The model under review builds one solid part; all positions refer to its coordinate system, in mm. A direction names the side the tool comes from. Give positions to 0.01 mm unless a question says otherwise; leave off trailing zeros. Order: outer loops, then holes, each group sorted by start corner. A loop starts at its lowest first (then second) coordinate and runs counter-clockwise, first axis right, second up. Notation, with made-up numbers: (21.5, 21) - (72.5, 21) arc R26 cw to (72.5, 50) - close; hole circle Ø4 at (65, 9). An arc over 180 degrees is marked (long way). Put each result on its own line as item: value.
```python
from build123d import *

# Parameters (mm, degrees)
CROQUIS1_R              = 25
SALIENTE_EXTRUIR1_DEPTH = 3
CROQUIS2_W              = 12.95
CROQUIS2_H              = 12.95
SALIENTE_EXTRUIR2_DEPTH = 3
CROQUIS3_R              = 2
CORTAR_EXTRUIR1_DEPTH   = 124.455998815
CROQUIS4_R              = 1.5
CORTAR_EXTRUIR2_DEPTH   = 124.455998815


with BuildPart() as part:
    # Croquis1 → Saliente-Extruir1 (new body)
    with BuildSketch(Plane.XY):
        with BuildLine():
            Line((-15.070986718, 74.306476298), (-15.070986718, 37.256476298))
            ThreePointArc((-15.070986718, 37.256476298), (-28.445175059, 28.391049341), (-37.285113206, 15))
            Line((-37.285113206, 15), (-74.335113206, 15))
            Line((-74.335113206, 15), (-74.335113206, 20.59))
            Line((-74.335113206, 20.59), (-87.285113206, 20.59))
            Line((-87.285113206, 20.59), (-87.285113206, -20.59))
            Line((-87.285113206, -20.59), (-74.335113206, -20.59))
            Line((-74.335113206, -20.59), (-74.335113206, -15))
            Line((-74.335113206, -15), (-37.285113206, -15))
            ThreePointArc((-37.285113206, -15), (-28.445175059, -28.391049341), (-15.070986718, -37.256476298))
            Line((-15.070986718, -37.256476298), (-15.070986718, -74.306476298))
            Line((-15.070986718, -74.306476298), (-20.660986718, -74.306476298))
            Line((-20.660986718, -74.306476298), (-20.660986718, -87.256476298))
            Line((-20.660986718, -87.256476298), (20.519013282, -87.256476298))
            Line((20.519013282, -87.256476298), (20.519013282, -74.306476298))
            Line((20.519013282, -74.306476298), (14.929013282, -74.306476298))
            Line((14.929013282, -74.306476298), (14.929013282, -37.256476298))
            ThreePointArc((14.929013282, -37.256476298), (28.353570497, -28.407666286), (37.22795272, -15))
            Line((37.22795272, -15), (59.27795272, -15))
            Line((59.27795272, -15), (59.27795272, -20.59))
            Line((59.27795272, -20.59), (72.22795272, -20.59))
            Line((72.22795272, -20.59), (72.22795272, 20.59))
            Line((72.22795272, 20.59), (59.27795272, 20.59))
            Line((59.27795272, 20.59), (59.27795272, 15))
            Line((59.27795272, 15), (37.22795272, 15))
            ThreePointArc((37.22795272, 15), (28.353570497, 28.407666286), (14.929013282, 37.256476298))
            Line((14.929013282, 37.256476298), (14.929013282, 74.306476298))
            Line((14.929013282, 74.306476298), (20.519013282, 74.306476298))
            Line((20.519013282, 74.306476298), (20.519013282, 87.256476298))
            Line((20.519013282, 87.256476298), (-20.660986718, 87.256476298))
            Line((-20.660986718, 87.256476298), (-20.660986718, 74.306476298))
            Line((-20.660986718, 74.306476298), (-15.070986718, 74.306476298))
        make_face()
        Circle(CROQUIS1_R, mode=Mode.SUBTRACT)
    extrude(amount=SALIENTE_EXTRUIR1_DEPTH)

    # Croquis2 → Saliente-Extruir2 (add)
    with BuildSketch(Plane(origin=(0, 0, 0), x_dir=(-1, 0, 0), z_dir=(0, 0, -1))):
        with Locations((-26.994013282, 80.781476298)):
            Rectangle(CROQUIS2_W, CROQUIS2_H)
        with Locations((27.135986718, 80.781476298)):
            Rectangle(CROQUIS2_W, CROQUIS2_H)
        with Locations((-26.994013282, -80.781476298)):
            Rectangle(CROQUIS2_W, CROQUIS2_H)
        with Locations((27.135986718, -80.781476298)):
            Rectangle(CROQUIS2_W, CROQUIS2_H)
        with Locations((80.810113206, 27.065)):
            Rectangle(CROQUIS2_W, CROQUIS2_H)
        with Locations((80.810113206, -27.065)):
            Rectangle(CROQUIS2_W, CROQUIS2_H)
    extrude(amount=-SALIENTE_EXTRUIR2_DEPTH)

    # Croquis3 → Cortar-Extruir1 (cut, through all)
    with BuildSketch(Plane(origin=(0, 0, 0), x_dir=(-1, 0, 0), z_dir=(0, 0, -1))):
        with Locations((-26.994013282, 80.781476298)):
            Circle(CROQUIS3_R)
        with Locations((27.135986718, 80.781476298)):
            Circle(CROQUIS3_R)
        with Locations((27.135986718, -80.781476298)):
            Circle(CROQUIS3_R)
        with Locations((-26.994013282, -80.781476298)):
            Circle(CROQUIS3_R)
        with Locations((80.810113206, -27.065)):
            Circle(CROQUIS3_R)
        with Locations((80.810113206, 27.065)):
            Circle(CROQUIS3_R)
    extrude(amount=-CORTAR_EXTRUIR1_DEPTH, mode=Mode.SUBTRACT)

    # Croquis4 → Cortar-Extruir2 (cut, through all)
    with BuildSketch(Plane(origin=(0, 0, 0), x_dir=(-1, 0, 0), z_dir=(0, 0, -1))):
        with Locations((-18.019013282, -84.756476298)):
            Circle(CROQUIS4_R)
        with Locations((-18.019013282, -76.806476298)):
            Circle(CROQUIS4_R)
        with Locations((18.160986718, -76.806476298)):
            Circle(CROQUIS4_R)
        with Locations((18.160986718, -84.756476298)):
            Circle(CROQUIS4_R)
        with Locations(Location((18.160986718, 76.806476298, 0), (0, 0, 180))):
            Circle(CROQUIS4_R)
        with Locations(Location((18.160986718, 84.756476298, 0), (0, 0, 180))):
            Circle(CROQUIS4_R)
        with Locations(Location((-18.019013282, 84.756476298, 0), (0, 0, 180))):
            Circle(CROQUIS4_R)
        with Locations(Location((-18.019013282, 76.806476298, 0), (0, 0, 180))):
            Circle(CROQUIS4_R)
        with Locations((76.835113206, -18.09)):
            Circle(CROQUIS4_R)
        with Locations(Location((84.785113206, -18.09, 0), (0, 0, 180))):
            Circle(CROQUIS4_R)
        with Locations(Location((76.835113206, 18.09, 0), (0, 0, 180))):
            Circle(CROQUIS4_R)
        with Locations((84.785113206, 18.09)):
            Circle(CROQUIS4_R)
        with Locations((-69.72795272, -18.09)):
            Circle(CROQUIS4_R)
        with Locations(Location((-61.77795272, -18.09, 0), (0, 0, 180))):
            Circle(CROQUIS4_R)
        with Locations(Location((-69.72795272, 18.09, 0), (0, 0, 180))):
            Circle(CROQUIS4_R)
        with Locations((-61.77795272, 18.09)):
            Circle(CROQUIS4_R)
    extrude(amount=-CORTAR_EXTRUIR2_DEPTH, mode=Mode.SUBTRACT)


solid = part.part
```
(1) Wall thickness on L1, parallel to Y at x = 32.5, z = 1.35; L2, parallel to Y at x = 23, z = 2.7; L3, parallel to Y at x = -20, z = 1.6: over which ranges is each line inside the solid? List them lowest first.
The answers:
L1: -87.26 to -74.31, -23.55 to 23.55, 74.31 to 87.26
L2: -87.26 to -74.31, -32.89 to -9.8, 9.8 to 32.89, 74.31 to 87.26
L3: -87.26 to -74.31, -34.86 to -15, 15 to 34.86, 74.31 to 87.26
(2) Take a section at C-C, the plane y = 65.5. Write out the cut boundary in (x, z).
The answers:
outline: (-15.07, 0) - (14.93, 0) - (14.93, 3) - (-15.07, 3) - close
(3) Clearance check with flat-ended pins moving along their axes: pin 1 Ø0.9 at (y, z) = (-81.5, 2) entering from +X; pin 2 Ø10 at (x, y) = (0, 57.5) entering from -Z; pin 3 Ø1.5 at (y, z) = (-81.5, 1) entering from -X; pin 4 Ø0.9 at (x, z) = (-48.5, 1.5) entering from -Y. State where each tip first meets the part, or that it passes through.
The answers:
pin 1: x = 33.47
pin 2: z = 0
pin 3: x = -33.61
pin 4: y = -15
(4) For faces 3 (the flat face through (-19, 20, 3)), 4 (the cylindrical face through (28.19, -28.57, 1.48)), list the 3-axis set-ups (+Z, -Z, +X, -X, +Y, -Y) from which the entire face can be reached by the end or side of a thin tool; tool diameter is ignored.
The answers:
face 3: +Z, +X, -X, +Y, -Y
face 4: +Z, -Z
(5) Take a section at A-A, the plane x = 0. Write out the cut boundary in (y, z), then the cut area to 3 significant figures.
The answers:
outline: (-87.26, 0) - (-25, 0) - (-25, 3) - (-87.26, 3) - close; (25, 0) - (87.26, 0) - (87.26, 3) - (25, 3) - close
area: 374 mm^2
(6) Take a section at B-B, the plane y = 0. Write out the cut boundary in (x, z).
The answers:
outline: (-87.29, 0) - (-25, 0) - (-25, 3) - (-87.29, 3) - close; (25, 0) - (72.23, 0) - (72.23, 3) - (25, 3) - close
(7) The part is to be moulded in two halves that separate along Y. For faces 1 (the cylindrical face through (-82.66, 26.3, 1.48)), 2 (the flat face through (-19, 20, 0)), say which applies: pulls with the +Y half, pulls with the -Y half, needs draft (parallel to the pull), parting line crosses it, or undercut.
The answers:
face 1: undercut
face 2: needs draft
(8) Take a section at D-D, the plane x = -61. Write out the cut boundary in (y, z).
The answers:
outline: (-15, 0) - (15, 0) - (15, 3) - (-15, 3) - close
